Could you check a few things on this model? Use its own coordinates, in mm. Give positions to 0.01 mm unless a question says otherwise; leave off trailing zeros. Order: outer loops, then holes, each group sorted by start corner. A loop starts at its lowest first (then second) coordinate and runs counter-clockwise, first axis right, second up.
(1) Imagine slicing it at A-A, the plane y = 1.8. Write out the boundary of the cut face in (x, z).
(2) Will this pin go through, and if not, where does the flat tip stop? pin 1 (3 mm diameter, centred on x = 31.77, z = -31.77, fed in from -Y).
(3) If I drill on probe 1 along X at (y, z) = (2.4, -32); probe 2 along X at (y, z) = (2.1, 32); probe 3 along X at (y, z) = (0.5, -30.5), over which ranges is the centre line in solid material (lowest first)?
(4) Imagine slicing it at B-B, the plane z = 26. Write out the boundary of the cut face in (x, y), then the cut area to 3 significant figures.
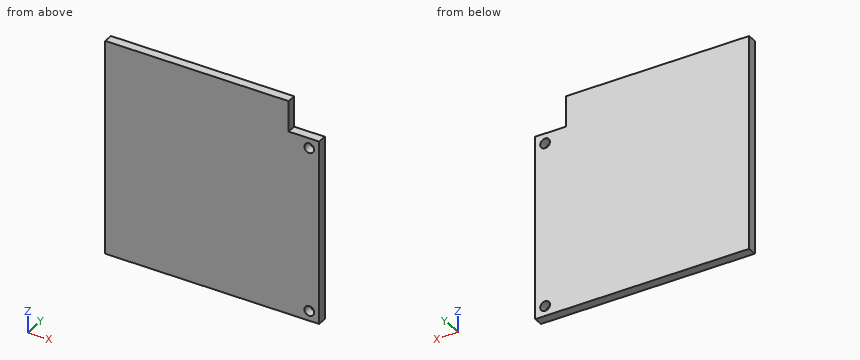
Autodesk Inventor part; units mm, degrees
ref_plane "YZ Plane" through (0, 0, 0) normal (1, 0, 0) x (0, 1, 0)
ref_plane "XZ Plane" through (0, 0, 0) normal (0, 1, 0) x (-1, 0, 0)
ref_plane "XY Plane" through (0, 0, 0) normal (0, 0, 1) x (1, 0, 0)
sketch "Эскиз1" plane through (0, 0, 0) normal (0, 1, 0) x (-1, 0, 0)
  line L0 (-35, 35) -> (35, 35)
  line L1 (35, 35) -> (35, -35)
  line L2 (35, -35) -> (-35, -35)
  line L3 (-35, -35) -> (-35, 35)
  line L4 (-35, 35) -> (35, -35) construction
  line L5 (35, 35) -> (-35, -35) construction
  line L6 (-35, 35) -> (-25, 35)
  line L7 (-25, 35) -> (-25, 25)
  line L8 (-25, 25) -> (-35, 25)
  line L9 (-35, 25) -> (-35, 35)
  circle A0 centre (-31.7678, 21.7678) radius 1.6
  line L10 (-35, -35) -> (-31.7678, -31.7678)
  circle A1 centre (-31.7678, -31.7678) radius 1.6
  point P0 (0, 0)
  point P1 (-35, 15)
  dimension "d0" = 70
  dimension "d1" = 70
  dimension "d3" = 10
  dimension "d5" = 3.2
  dimension "d7" = 4.571
  dimension "d8" = 3.2
  dimension "d11" = 4.5711
  dimension "d12" = 10
extrude "Выдавливание1" add sketch "Эскиз1" along normal blind 3 contours L0 L1 L2 L3 L8 L7
properties part number "000.109 - Правая боковая панель заднего сегмента"
Answer block:
1. outline: (-35, -35) - (35, -35) - (35, 25) - (25, 25) - (25, 35) - (-35, 35) - close; hole circle Ø3.2 at (31.77, -31.77); hole circle Ø3.2 at (31.77, 21.77)
2. pin 1: passes through
3. probe 1: x = -35 to 30.18, 33.35 to 35
3. probe 2: x = -35 to 25
3. probe 3: x = -35 to 30.79, 32.74 to 35
4. outline: (-35, 0) - (25, 0) - (25, 3) - (-35, 3) - close
4. area: 180 mm2
